from build123d import *

# Parameters (mm, degrees)
SKETCH1_R           = 5
BOSS_EXTRUDE1_DEPTH = 1
SKETCH2_R           = 4
BOSS_EXTRUDE2_DEPTH = 3
SKETCH3_R           = 1.5
CUT_EXTRUDE1_DEPTH  = 13


with BuildPart() as part:
    # Sketch1 → Boss-Extrude1 (new body)
    with BuildSketch(Plane(origin=(0, 0, 0), x_dir=(1, 0, 0), z_dir=(0, 1, 0))):
        Circle(SKETCH1_R)
    extrude(amount=BOSS_EXTRUDE1_DEPTH)

    # Sketch2 → Boss-Extrude2 (add)
    with BuildSketch(Plane.XZ):
        Circle(SKETCH2_R)
    extrude(amount=BOSS_EXTRUDE2_DEPTH)

    # Sketch3 → Cut-Extrude1 (cut)
    with BuildSketch(Plane.XZ.offset(3)):
        Circle(SKETCH3_R)
    extrude(amount=-CUT_EXTRUDE1_DEPTH, mode=Mode.SUBTRACT)


solid = part.part
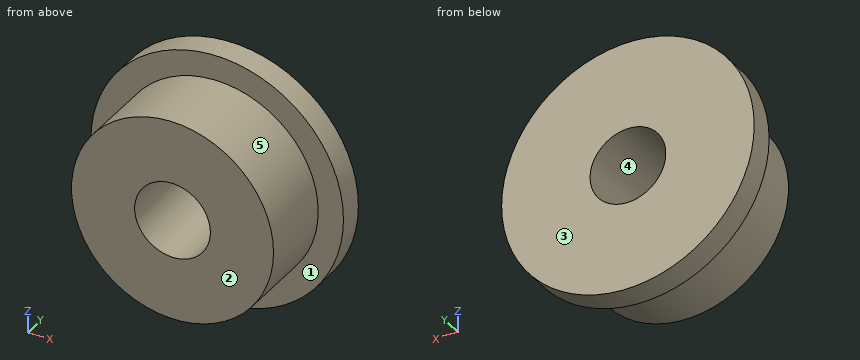
For this review, take the finished solid that the model builds, in its own axes (mm). Face numbers are marked on the shaded views. A direction names the side the tool comes from. Round coordinates to 2 decimals unless told otherwise and drop trailing zeros. Loops run counter-clockwise (first coordinate to the right, second up) from the corner with the lowest first, then second, coordinate; pieces in that order, holes last. Notation, with made-up numbers: (-30.5, 28) - (-16.5, 28) arc R6 ccw to (-16.5, 33) - close; hole circle Ø4 at (19.5, 3). An arc over 180 degrees is marked (long way). One line per question, with ' | ' between items.
Q1. Take a section at A-A (z = 0). Give the boundary of the cut face in (x, y), and give its area (3 significant figures).
Taken from the geometry:
outline: (-5, 0) - (-4, 0) - (-4, -3) - (-1.5, -3) - (-1.5, 1) - (-5, 1) - close; (1.5, -3) - (4, -3) - (4, 0) - (5, 0) - (5, 1) - (1.5, 1) - close | area: 22.0 mm²
Q2. The part is to be moulded in two halves that separate along Z. For the marked faces 3, 4 and 5, say which applies: released by +Z, released by -Z, zero draft, split by the parting line, or undercut.
Taken from the geometry:
face 3: zero draft | face 4: undercut | face 5: split by the parting line
Q3. Take a section at B-B (x = 0). Give the boundary of the cut face in (y, z).
Taken from the geometry:
outline: (-3, -4) - (0, -4) - (0, -5) - (1, -5) - (1, -1.5) - (-3, -1.5) - close; (-3, 1.5) - (1, 1.5) - (1, 5) - (0, 5) - (0, 4) - (-3, 4) - close
Q4. Take a section at D-D (z = -1.75). Give the boundary of the cut face in (x, y).
Taken from the geometry:
outline: (-4.68, 0) - (-3.6, 0) - (-3.6, -3) - (3.6, -3) - (3.6, 0) - (4.68, 0) - (4.68, 1) - (-4.68, 1) - close
Q5. Tool access review of the marked faces 1 and 2: name each direction out of +Z, -Z, +X, -X, +Y, -Y from which nothing blocks a thin tool from reaching the whole face with its end or side.
Taken from the geometry:
face 1: -Y | face 2: +Z, -Z, +X, -X, -Y
Q6. Take a section at C-C (y = 0.4). Give the boundary of the cut face in (x, z).
Taken from the geometry:
outline: circle Ø10 at (0, 0); hole circle Ø3 at (0, 0)
Q7. For line 1 along Z through (x, y) = (0, -1.2); line 2 along Y through (x, z) = (2.5, -3.75); line 3 along X through (y, z) = (-0.85, 0.25), list the stretches that pass through material, from the lowest coordinate up. Write a range as [from, to].
Taken from the geometry:
line 1: z = [-4, -1.5], [1.5, 4] | line 2: y = [0, 1] | line 3: x = [-3.99, -1.48], [1.48, 3.99]
